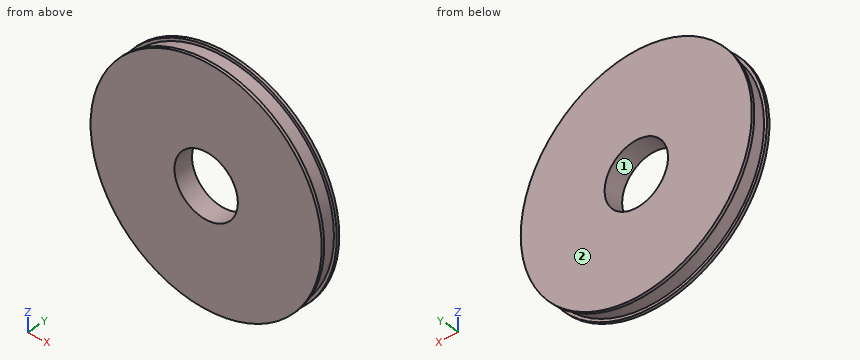
Autodesk Inventor part; units mm, degrees
ref_plane "YZ Plane" through (0, 0, 0) normal (1, 0, 0) x (0, 1, 0)
ref_plane "XZ Plane" through (0, 0, 0) normal (0, 1, 0) x (-1, 0, 0)
ref_plane "XY Plane" through (0, 0, 0) normal (0, 0, 1) x (1, 0, 0)
sketch "Skizze1" plane through (0, 0, 0) normal (0, 1, 0) x (-1, 0, 0)
  circle A0 centre (0, 0) radius 80
  dimension "d0" = 160
extrude "Extrusion1" add sketch "Skizze1" along normal blind 10
sketch "Skizze2" plane through (0, 10, 0) normal (0, 1, 0) x (1, 0, 0)
  circle A0 centre (0, 0) radius 82
  dimension "d3" = 164
extrude "Extrusion2" add sketch "Skizze2" along normal blind 2
sketch "Skizze3" plane through (0, 0, 0) normal (0, -1, 0) x (1, 0, 0)
  circle A0 centre (0, 0) radius 82
  dimension "d6" = 164
extrude "Extrusion3" add sketch "Skizze3" along normal blind 2
sketch "Skizze4" plane through (0, -2, 0) normal (0, -1, 0) x (1, 0, 0)
  circle A0 centre (0, 0) radius 22.5
  dimension "d9" = 45
extrude "Extrusion4" cut sketch "Skizze4" against normal blind 14
properties part number "Antriebsscheibe"
For this review, take the finished solid that the model builds, in its own axes (mm). Face numbers are marked on the shaded views. Round coordinates to 2 decimals unless told otherwise and drop trailing zeros. Write each loop counter-clockwise with the first axis right and the second up, starting at its lowest first coordinate (ties: lowest second). Pieces come first, ordered by that corner, then holes. Notation, with made-up numbers: M 20.25,49.5 L 79.25,49.5 A16 ccw 79.25,67.5 Z; hole C 4.25,40.25 d9. An arc over 180 degrees is marked long. Write item = value, one per line. Start each with the question number.
(1) Clearance check with flat-ended pins moving along their axes: pin 1 Ø4 at (x, y) = (14, 4.5) entering from -Z; pin 2 Ø2 at (x, z) = (21, 4) entering from -Y; pin 3 Ø3 at (y, z) = (5, 23) entering from +X; pin 4 Ø4 at (x, y) = (-8, 6.5) entering from +Z. State where each tip first meets the part, or that it passes through.
(2) We need section D-D (x = -34). Give the boundary of the cut face in (y, z), then the cut area to 3 significant figures.
(3) For line 1 along Z through (x, y) = (0, 3.75); line 2 along Z through (x, y) = (-5, 9.75); line 3 along X through (y, z) = (9.75, -20.5), list the stretches that pass through material, from the lowest coordinate up.
(4) We need section A-A (x = 0). Give the boundary of the cut face in (y, z), then the cut area to 3 significant figures.
(5) We need section B-B (z = 0). Give the boundary of the cut face in (x, y), then the cut area to 3 significant figures.
(6) The part is to be moulded in two halves that separate along Z. For the marked faces 1 and 2, say which applies: +Z half, -Z half, draft (parallel to the pull), parting line (faces both ways), or undercut.
(7) We need section C-C (y = 4). Give the boundary of the cut face in (x, z).
Results found:
q1.pin_1 = -79.09
q1.pin_2 = through
q1.pin_3 = 77.06
q1.pin_4 = 79.77
q2.outline = M -2,-74.62 L 0,-74.62 L 0,-72.42 L 10,-72.42 L 10,-74.62 L 12,-74.62 L 12,74.62 L 10,74.62 L 10,72.42 L 0,72.42 L 0,74.62 L -2,74.62 Z
q2.area = 2,050 mm²
q3.line_1 = -80 to -22.5, 22.5 to 80
q3.line_2 = -79.84 to -21.94, 21.94 to 79.84
q3.line_3 = -77.33 to -9.27, 9.27 to 77.33
q4.outline = M -2,-82 L 0,-82 L 0,-80 L 10,-80 L 10,-82 L 12,-82 L 12,-22.5 L -2,-22.5 Z; M -2,22.5 L 12,22.5 L 12,82 L 10,82 L 10,80 L 0,80 L 0,82 L -2,82 Z
q4.area = 1,630 mm²
q5.outline = M -82,-2 L -22.5,-2 L -22.5,12 L -82,12 L -82,10 L -80,10 L -80,0 L -82,0 Z; M 22.5,-2 L 82,-2 L 82,0 L 80,0 L 80,10 L 82,10 L 82,12 L 22.5,12 Z
q5.area = 1,630 mm²
q6.face_1 = undercut
q6.face_2 = draft
q7.outline = C 0,0 d160; hole C 0,0 d45
